Input: part model. Units: mm. Frame: model coordinates. Face numbers are marked on the shaded views. A direction names the side the tool comes from. Coordinates: 2 decimals unless noted, no trailing zeros. Order: outer loops, then holes, each group sorted by start corner. A loop starts at its lowest first (then second) coordinate and runs counter-clockwise, first axis right, second up. Notation, with made-up numbers: (50.5, 45) -> (75.5, 45) arc R25 cw to (75.5, 74) -> close; hole circle Ø3 at (74.25, 15.5). An arc over 180 degrees is marked (long way). One line per question, with ' | ' between items.
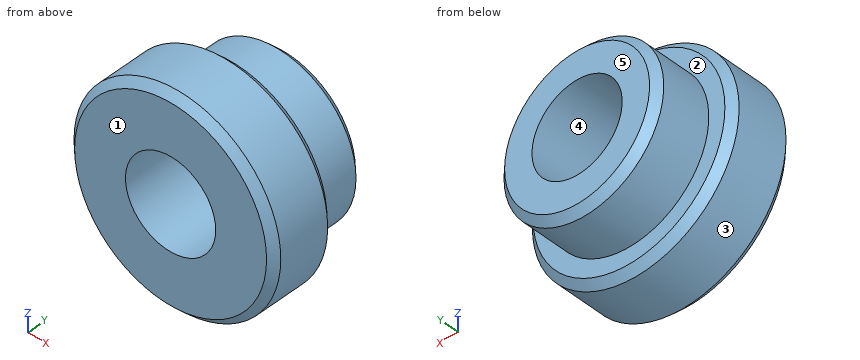
```python
from build123d import *

# Parameters (mm, degrees)
SKETCH1_R           = 2.794
BOSS_EXTRUDE1_DEPTH = 1.778
CHAMFER1_SIZE       = 0.2
SKETCH2_R           = 2.159
BOSS_EXTRUDE2_DEPTH = 1.524
CHAMFER2_SIZE       = 0.2
SKETCH3_R           = 1.2192
CUT_EXTRUDE1_DEPTH  = 4.302


with BuildPart() as part:
    # Sketch1 → Boss-Extrude1 (new body)
    with BuildSketch(Plane(origin=(0, 0, 0), x_dir=(1, 0, 0), z_dir=(0, 1, 0))):
        Circle(SKETCH1_R)
    extrude(amount=BOSS_EXTRUDE1_DEPTH)

    # Chamfer1
    chamfer1_edges = [part.edges().sort_by_distance(p)[0] for p in [
        (-2.794, 0, 0),
        (-2.794, 1.778, 0),
    ]]
    chamfer(chamfer1_edges, length=CHAMFER1_SIZE)

    # Sketch2 → Boss-Extrude2 (add)
    with BuildSketch(Plane(origin=(0, 1.778, 0), x_dir=(1, 0, 0), z_dir=(0, 1, 0))):
        Circle(SKETCH2_R)
    extrude(amount=BOSS_EXTRUDE2_DEPTH)

    # Chamfer2
    chamfer2_edges = [part.edges().sort_by_distance(p)[0] for p in [
        (-2.159, 3.302, 0),
    ]]
    chamfer(chamfer2_edges, length=CHAMFER2_SIZE)

    # Sketch3 → Cut-Extrude1 (cut, through all)
    with BuildSketch(Plane(origin=(0, 3.302, 0), x_dir=(1, 0, 0), z_dir=(0, 1, 0))):
        Circle(SKETCH3_R)
    extrude(amount=-CUT_EXTRUDE1_DEPTH, mode=Mode.SUBTRACT)


solid = part.part
```
1. Pin query (flat end, axial travel): pin 1 Ø1 at (x, y) = (-1.5, 3) entering from +Z. Return the tip coordinate at first contact, or that it passes through.
Recorded:
pin 1: stops at z = 1.91
2. Cut plane B-B, the plane z = 0. Return loops of the section in (x, y).
Recorded:
outline: (-2.79, 0.2) -> (-2.59, 0) -> (-1.22, 0) -> (-1.22, 3.3) -> (-1.96, 3.3) -> (-2.16, 3.1) -> (-2.16, 1.78) -> (-2.59, 1.78) -> (-2.79, 1.58) -> close; (1.22, 0) -> (2.59, 0) -> (2.79, 0.2) -> (2.79, 1.58) -> (2.59, 1.78) -> (2.16, 1.78) -> (2.16, 3.1) -> (1.96, 3.3) -> (1.22, 3.3) -> close
3. Access query for the marked faces 1 and 2. Directions: +Z, -Z, +X, -X, +Y, -Y. A direction counts if a zero-diameter tool reaches every point of the face in a straight line with its end or side. Return the directions, or none.
Recorded:
face 1: +Z, -Z, +X, -X, -Y | face 2: +Y
4. Ray query, line 1 (Z direction, x = 0, y = 1.4); line 2 (X direction, y = 1.85, z = 0). Return the intervals inside material, ascending. Write a range as [from, to].
Recorded:
line 1: z = [-2.79, -1.22], [1.22, 2.79] | line 2: x = [-2.16, -1.22], [1.22, 2.16]
5. Cut plane D-D, the plane y = 2.65. Return loops of the section in (x, z).
Recorded:
outline: circle Ø4.32 at (0, 0); hole circle Ø2.44 at (0, 0)
6. Mould query, pull axis Z, two halves, no side actions, for the marked faces 3, 4 and 5. Classes: released by +Z, released by -Z, zero draft, split by the parting line, or undercut.
Recorded:
face 3: split by the parting line | face 4: undercut | face 5: zero draft
7. Cut plane A-A, the plane x = 0. Return loops of the section in (y, z).
Recorded:
outline: (0, -2.59) -> (0.2, -2.79) -> (1.58, -2.79) -> (1.78, -2.59) -> (1.78, -2.16) -> (3.1, -2.16) -> (3.3, -1.96) -> (3.3, -1.22) -> (0, -1.22) -> close; (0, 1.22) -> (3.3, 1.22) -> (3.3, 1.96) -> (3.1, 2.16) -> (1.78, 2.16) -> (1.78, 2.59) -> (1.58, 2.79) -> (0.2, 2.79) -> (0, 2.59) -> close
8. Cut plane C-C, the plane y = 1.05. Return loops of the section in (x, z).
Recorded:
outline: circle Ø5.59 at (0, 0); hole circle Ø2.44 at (0, 0)
